Autodesk Inventor part; units mm, degrees
ref_plane "YZ Plane" through (0, 0, 0) normal (1, 0, 0) x (0, 1, 0)
ref_plane "XZ Plane" through (0, 0, 0) normal (0, 1, 0) x (-1, 0, 0)
ref_plane "XY Plane" through (0, 0, 0) normal (0, 0, 1) x (1, 0, 0)
sketch "Sketch1" plane through (0, 0, 0) normal (0, 1, 0) x (-1, 0, 0)
  line L0 (-34.98, 44.98) -> (34.98, 44.98)
  line L1 (34.98, 44.98) -> (34.98, -44.98)
  line L2 (34.98, -44.98) -> (-34.98, -44.98)
  line L3 (-34.98, -44.98) -> (-34.98, 44.98)
  line L4 (-34.98, 44.98) -> (34.98, -44.98) construction
  line L5 (34.98, 44.98) -> (-34.98, -44.98) construction
  point P0 (0, 0)
  dimension "d0" = 89.96
  dimension "d1" = 69.96
extrude "Extrusion1" add sketch "Sketch1" along normal blind 10
sketch "Sketch2" plane through (0, 10, 0) normal (0, 1, 0) x (1, 0, 0)
  circle A0 centre (10, 28.2843) radius 7.52
  line L0 (-34.98, 44.98) -> (-34.98, -44.98)
  point P0 (0, 0)
  dimension "d4" = 30
  dimension "d5" = 15.04
  dimension "d6" = 44.98
sketch "Sketch3" plane through (0, 10, 0) normal (0, 1, 0) x (1, 0, 0)
  line L0 (24.02, -38.04) -> (-24.02, -38.04)
  line L1 (-24.02, -38.04) -> (-24.02, 12)
  line L2 (-24.02, 12) -> (24.02, 12)
  line L3 (24.02, 12) -> (24.02, -38.04)
  line L4 (24.02, -38.04) -> (-24.02, 12) construction
  line L5 (-24.02, -38.04) -> (24.02, 12) construction
  point P0 (0, 0)
  point P1 (0, -13.02)
  dimension "d9" = 12
  dimension "d10" = 50.04
  dimension "d11" = 48.04
  dimension "d12" = 0
extrude "Extrusion3" cut sketch "Sketch3" against normal blind 5.04
extrude "Extrusion4" cut sketch "Sketch2" against normal through all
sketch "Sketch6" plane through (-34.98, 0, 44.98) normal (0, 0, 1) x (1, 0, 0)
  line L0 (39.98, 5) -> (49.98, 5)
  line L1 (49.98, 5) -> (49.98, 15)
  line L2 (49.98, 15) -> (39.98, 15)
  line L3 (39.98, 15) -> (39.98, 5)
  line L4 (37.46, 10) -> (52.5, 10)
  line L5 (39.98, 5) -> (49.98, 15) construction
  line L6 (49.98, 5) -> (39.98, 15) construction
  point P0 (34.98, 0)
  point P1 (44.98, 10)
  dimension "d29" = 10
  dimension "d30" = 10
extrude "Extrusion5" cut sketch "Sketch6" against normal blind 33
sketch "Sketch7" plane through (0, 10, 0) normal (0, 1, 0) x (1, 0, 0)
  circle A0 centre (10, 28.2843) radius 7.52
  circle A1 centre (10, 35.8043) radius 5
  circle A2 centre (10, 20.7643) radius 5
  point P0 (0, 0)
  dimension "d34" = 10
  dimension "d35" = 10
  dimension "d36" = 15.04
coil "Coil2" sketch "Sketch7" operation add axis through (0, -10, 0) along (0, -1, 0) pitch 50 turns 0.2 hand left contours A2 A0 | A0 A2
sketch "Sketch8" plane through (0, 10, 0) normal (0, 1, 0) x (1, 0, 0)
  arc A0 (14.7156, 22.4265) -> (5.2844, 22.4265) centre (10, 28.2843) ccw
  circle A1 centre (10, 35.8043) radius 5
  point P0 (0, 0)
  point P1 (10, 35.8043)
  dimension "d45" = 10
coil "Coil3" sketch "Sketch8" operation add axis through (0, -10, 0) along (0, -1, 0) pitch 50 turns 0.2 hand right
sketch "Sketch9" plane through (34.98, 0, -44.98) normal (1, 0, 0) x (0, 0, -1)
  line L0 (-89.96, 10) -> (0, 10)
  line L1 (0, 0) -> (-38.9181, 0)
  line L2 (-89.96, 10) -> (0, 10)
  line L3 (0, 10) -> (0, 0)
  line L4 (0, 0) -> (-89.96, 0)
  line L5 (-89.96, 0) -> (-89.96, 10)
  point P0 (-44.98, 0)
extrude "Extrusion6" cut sketch "Sketch9" along normal blind 20
For this review, take the finished solid that the model builds, in its own axes (mm). A direction names the side the tool comes from. Round coordinates to 2 decimals unless told otherwise and drop trailing zeros. Order: outer loops, then holes, each group sorted by start corner. A loop starts at its lowest first (then second) coordinate and runs counter-clockwise, first axis right, second up. Notation, with made-up numbers: (76.25, 33) -> (108.25, 33) arc R35 ccw to (108.25, 68) -> close; hole circle Ø1 at (67, -18.5). An arc over 180 degrees is marked (long way). Use a Markdown table: item, result.
Item 1: For line 1 along Z through (x, y) = (10, 3.25); line 2 along X through (y, z) = (5.5, 34); line 3 along Z through (x, y) = (-14, 7.5), list the stretches that pass through material, from the lowest coordinate up. Write a range as [from, to].
Resolved:
| item | result |
|---|---|
| line 1 | z = [-44.98, -35.8], [-20.76, 44.98] |
| line 2 | x = [-34.98, -24.02], [24.02, 34.98] |
| line 3 | z = [-44.98, -12], [38.04, 44.98] |
Item 2: For pin 1 (7.5 mm diameter, centred on x = 9.5, z = 40.5, fed in from +Y); pin 2 (9 mm diameter, centred on x = 10, z = -28.28, fed in from -Y), all flat-tipped, find the tip position at first contact; note any pin that passes through.
Resolved:
| item | result |
|---|---|
| pin 1 | stops at y = 5 |
| pin 2 | stops at y = 7.17 |
Item 3: Draft analysis for pull direction X (two halves, no side actions). For faces 4 (the flat face through (34.98, 5, -1)), 5 (the flat face through (5, 8, 42)), 6 (the flat face through (0, 0, 1)), state which applies: +X half, -X half, draft (parallel to the pull), parting line (faces both ways), or undercut.
Resolved:
| item | result |
|---|---|
| face 4 | +X half |
| face 5 | undercut |
| face 6 | draft |
Item 4: Take a section at A-A (z = 4). State the section outline as (x, y) points, plus the area to 3 significant figures.
Resolved:
| item | result |
|---|---|
| outline | (-34.98, 0) -> (34.98, 0) -> (34.98, 10) -> (24.02, 10) -> (24.02, 4.96) -> (-24.02, 4.96) -> (-24.02, 10) -> (-34.98, 10) -> close |
| area | 457 mm² |
Item 5: Machinability: for faces 1 (the flat face through (15, 7, 42)), 2 (the flat face through (-24.02, 8, 13)), 3 (the flat face through (-34.98, 5, 1)), which of the approach directions +Z, -Z, +X, -X, +Y, -Y give a long, thin tool a straight path to every point of the face, cutting with its end or side? Answer none if there is none.
Resolved:
| item | result |
|---|---|
| face 1 | +Z, +Y |
| face 2 | +Y |
| face 3 | +Z, -Z, -X, +Y, -Y |
Item 6: Take a section at B-B (x = -10). State the section outline as (y, z) points.
Resolved:
| item | result |
|---|---|
| outline | (0, -44.98) -> (10, -44.98) -> (10, -12) -> (4.96, -12) -> (4.96, 38.04) -> (10, 38.04) -> (10, 44.98) -> (0, 44.98) -> close |
